The model under review builds one solid part; all positions refer to its coordinate system, in mm. Face numbers are marked on the shaded views. Coordinates: 2 decimals unless noted, no trailing zeros. Write each loop counter-clockwise with the first axis right and the second up, starting at its lowest first coordinate (ties: lowest second). Pieces come first, ordered by that corner, then holes.
```python
from build123d import *

# Parameters (mm, degrees)
SKETCH2_W           = 30
SKETCH2_H           = 52
BOSS_EXTRUDE1_DEPTH = 2
SKETCH2_3_W         = 34.4
SKETCH2_3_H         = 56.4
SKETCH2_3_W_2       = 30
SKETCH2_3_H_2       = 52
BOSS_EXTRUDE2_DEPTH = 5
SKETCH3_W           = 28.685719202
SKETCH3_H           = 4.374860236
CUT_EXTRUDE1_DEPTH  = 6


with BuildPart() as part:
    # Sketch2 → Boss-Extrude1 (new body)
    with BuildSketch(Plane(origin=(0, 0, 0), x_dir=(1, 0, 0), z_dir=(0, 1, 0))):
        Rectangle(SKETCH2_W, SKETCH2_H)
    extrude(amount=BOSS_EXTRUDE1_DEPTH)

    # Sketch2<3> → Boss-Extrude2 (add)
    with BuildSketch(Plane(origin=(0, 0, 0), x_dir=(1, 0, 0), z_dir=(0, 1, 0))):
        Rectangle(SKETCH2_3_W, SKETCH2_3_H)
        Rectangle(SKETCH2_3_W_2, SKETCH2_3_H_2, mode=Mode.SUBTRACT)
    extrude(amount=BOSS_EXTRUDE2_DEPTH)

    # Sketch3 → Cut-Extrude1 (cut)
    with BuildSketch(Plane.XY.offset(28.2)):
        with Locations((-0.813326627, 3.719763482)):
            Rectangle(SKETCH3_W, SKETCH3_H)
    extrude(amount=-CUT_EXTRUDE1_DEPTH, mode=Mode.SUBTRACT)


solid = part.part
```
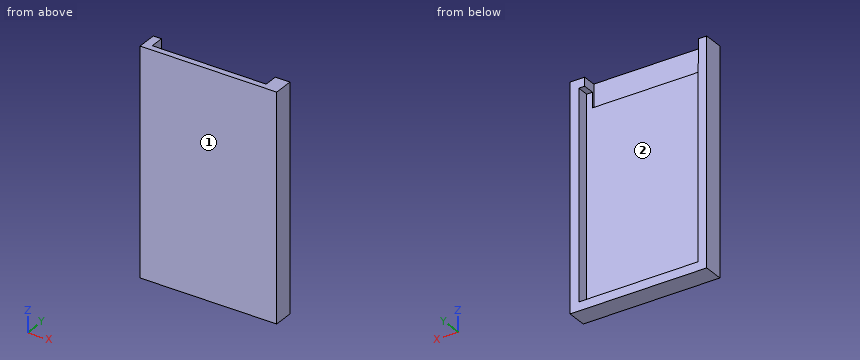
Item 1: Take a section at D-D, the plane z = -12. Write out the cut boundary in (x, y), plus the area to 3 significant figures.
Solved:
outline: (-17.2, 0) - (17.2, 0) - (17.2, 5) - (15, 5) - (15, 2) - (-15, 2) - (-15, 5) - (-17.2, 5) - close
area: 82.0 mm2
Item 2: Take a section at B-B, the plane z = 23. Write out the cut boundary in (x, y), plus the area to 3 significant figures.
Solved:
outline: (-17.2, 0) - (17.2, 0) - (17.2, 5) - (15, 5) - (15, 2) - (13.53, 2) - (13.53, 1.53) - (-15.16, 1.53) - (-15.16, 5) - (-17.2, 5) - close
area: 68.1 mm2
Item 3: For pin 1 (3 mm diameter, centred on x = 3, z = 26, fed in from +Y); pin 2 (1.5 mm diameter, centred on x = -7, y = 3.5, fed in from +Z); pin 3 (1 mm diameter, centred on x = -11.5, z = -9, fed in from -Y); pin 4 (1.7 mm diameter, centred on x = -1.5, y = 2.5, fed in from +Z), all flat-tipped, find the tip position at first contact; note any pin that passes through.
Solved:
pin 1: stops at y = 1.53
pin 2: stops at z = -26
pin 3: stops at y = 0
pin 4: stops at z = 22.2
Item 4: Take a section at C-C, the plane x = 11. Write out the cut boundary in (y, z).
Solved:
outline: (0, -28.2) - (5, -28.2) - (5, -26) - (2, -26) - (2, 22.2) - (1.53, 22.2) - (1.53, 28.2) - (0, 28.2) - close
Item 5: Take a section at A-A, the plane y = 2.65. Write out the cut boundary in (x, z).
Solved:
outline: (-17.2, -28.2) - (17.2, -28.2) - (17.2, 28.2) - (13.53, 28.2) - (13.53, 26) - (15, 26) - (15, -26) - (-15, -26) - (-15, 22.2) - (-15.16, 22.2) - (-15.16, 28.2) - (-17.2, 28.2) - close
Item 6: Mouldability with a two-part tool opening along X and no side actions: class the marked faces 1 and 2 as pulls with the +X half, pulls with the -X half, needs draft (parallel to the pull), parting line crosses it, or undercut.
Solved:
face 1: needs draft
face 2: undercut
Item 7: To check wall thickness, follow line 1 along X through (y, z) = (3.6, -6); line 2 along Z through (x, y) = (-6, 3.95); line 3 along X through (y, z) = (3.75, 25.5). State the ranges of each line that lie inside material, in increasing order.
Solved:
line 1: x = -17.2 to -15, 15 to 17.2
line 2: z = -28.2 to -26
line 3: x = -17.2 to -15.16, 15 to 17.2
